The listing builds one solid part. Answer for the finished solid, in the listing's coordinates (mm). A direction names the side the tool comes from. Round coordinates to 2 decimals unless told otherwise and drop trailing zeros. Answer as CSV lines item,"result". Start each with the question number.
from build123d import *

# Parameters (mm, degrees)
FILLET4_R          = 0.635
SKETCH10_R         = 4.0005
CUT_EXTRUDE5_DEPTH = 11.684
CUT_EXTRUDE6_DEPTH = 82.55


with BuildPart() as part:
    # Sketch9 → Revolve2 (revolve)
    with BuildSketch(Plane(origin=(0, 0, 0), x_dir=(0, 0, -1), z_dir=(1, 0, 0))):
        with BuildLine():
            Line((0, 0), (50.8, 0))
            ThreePointArc((50.8, 0), (28.251626652, 17.630503777), (0, 22.225))
            Line((0, 22.225), (0, 0))
        make_face()
    revolve(axis=Axis((0, 0, 0), (0, 0, -1)))

    # Fillet4
    fillet4_edges = [part.edges().sort_by_distance(p)[0] for p in [
        (0, -22.225, 0),
    ]]
    fillet(fillet4_edges, radius=FILLET4_R)

    # Sketch10 → Cut-Extrude5 (cut)
    with BuildSketch(Plane.XY):
        Circle(SKETCH10_R)
    extrude(amount=-CUT_EXTRUDE5_DEPTH, mode=Mode.SUBTRACT)

    # Sketch11 → Cut-Extrude6 (cut)
    with BuildSketch(Plane.XY):
        with BuildLine():
            Line((6.872643409, 1.269271981), (12.073562746, 1.269271981))
            ThreePointArc((12.073562746, 1.269271981), (13.327653654, 0.015181073), (12.073562746, -1.238909835))
            Line((12.073562746, -1.238909835), (6.872643409, -1.238909835))
            ThreePointArc((6.872643409, -1.238909835), (5.618552501, 0.015181073), (6.872643409, 1.269271981))
        make_face()
        with BuildLine():
            Line((-6.872643409, 1.269271981), (-12.073562746, 1.269271981))
            ThreePointArc((-12.073562746, 1.269271981), (-13.327653654, 0.015181073), (-12.073562746, -1.238909835))
            Line((-12.073562746, -1.238909835), (-6.872643409, -1.238909835))
            ThreePointArc((-6.872643409, -1.238909835), (-5.618552501, 0.015181073), (-6.872643409, 1.269271981))
        make_face()
    extrude(amount=-CUT_EXTRUDE6_DEPTH, mode=Mode.SUBTRACT)


solid = part.part
Q1. Straight lines are drawn through the part: L1, parallel to Y at x = 0, z = -7.5; L2, parallel to Y at x = 0, z = -5; L3, parallel to Z at x = 1, y = -18. For each, find the intervals that lie inside material, in ascending order.
Q2. For faces 1 (the face through (-0.9, -3.9, -5.8)), 2 (the face through (9, 1.269, -22)), determine the directions among +Z, -Z, +X, -X, +Y, -Y from which every point of the face is accessible in a straight line to the end or side of a thin tool.
Q3. Each of these flat-tipped pins is pushed along its axis until it touches: P1, Ø6, axis at y = -6.5, z = -42.5, coming from the +X side; P2, Ø1.6, axis at x = -9.5, z = -17, coming from the -Y side; P3, Ø1.5, axis at x = -3, z = -44.5, coming from the +Y side. Where does it stop, or does it pass through?
Q4. Find section A-A (z = -17). Count the separate pieces of the cut face and the enclosed holes in it, plus the area to 3 significant figures.
Q5. The mould has two halves that part along X. Classify faces 3 (the face through (-5, 0, 0)), 4 (the face through (-9, 1.269, -22)): +X half, -X half, draft (parallel to the pull), parting line (faces both ways), or undercut.
Reported:
1,L1,"y = -22.41 to -4, 4 to 22.41"
1,L2,"y = -22.46 to -4, 4 to 22.46"
1,L3,"z = -27.32 to 0"
2,face 1,"+Z"
2,face 2,"+Z, -Z"
3,P1,"stops at x = 9.58"
3,P2,"stops at y = -19.41"
3,P3,"stops at y = 7.07"
4,separate pieces,"1"
4,enclosed holes,"2"
4,area,"1,380 mm2"
5,face 3,"draft"
5,face 4,"undercut"
